Input: part model. Units: mm. Frame: model coordinates. A direction names the side the tool comes from. Round coordinates to 2 decimals unless told otherwise and drop trailing zeros. Loops run counter-clockwise (first coordinate to the right, second up) from the corner with the lowest first, then second, coordinate; pieces in that order, holes last.
1) Ray query, line 1 along Z through (x, y) = (6, 1) (3 decimals); line 2 along X through (y, z) = (2.45, -4). Return the intervals inside material, ascending.
2) Draft query along X for faces 1 (the face through (-14.676, 2.535, 12.768)), 2 (the face through (19.378, 2.535, -1.703)), 3 (the face through (1.792, 1.014, -4.858)). Return one class per face: pulls with the +X half, pulls with the -X half, needs draft (parallel to the pull), parting line crosses it, or undercut.
3) Section A-A, the plane z = 6. Return loops of the section in (x, y) (3 decimals), and give its area (3 significant figures).
4) First-contact query: pin 1 (3.5 mm diameter, centred on x = 0, z = 0, fed in from +Y); pin 2 (7 mm diameter, centred on x = -6, z = 0, fed in from +Y). Flat tips, straight axial feed; report the tip coordinate or a pass-through.
5) Access query for faces 4 (the face through (12.768, 2.535, 14.676)), 5 (the face through (7.55, 2.54, -17.87)), 6 (the face through (18.956, 2.535, 4.369)), 7 (the face through (-18.89, 2.54, 4.4)), 8 (the face through (-2.17, 3.52, 9.76)). Directions: +Z, -Z, +X, -X, +Y, -Y. A direction counts if a zero-diameter tool reaches every point of the face in a straight line with its end or side. Return the directions, or none.
6) Section C-C, the plane x = 16. Return loops of the section in (y, z), and give its area (3 significant figures).
7) Section B-B, the plane x = 6. Return loops of the section in (y, z) (3 decimals), and give its area (3 significant figures).
Autodesk Inventor part; units mm, degrees
ref_plane "YZ Plane" through (0, 0, 0) normal (1, 0, 0) x (0, 1, 0)
ref_plane "XZ Plane" through (0, 0, 0) normal (0, 1, 0) x (-1, 0, 0)
ref_plane "XY Plane" through (0, 0, 0) normal (0, 0, 1) x (1, 0, 0)
sketch "Sketch1" plane through (0, 0, 0) normal (0, 1, 0) x (-1, 0, 0)
  circle A0 centre (0, 0) radius 17.5
  dimension "d0" = 35
extrude "Extrusion1" add sketch "Sketch1" along normal blind 5
sketch "Sketch2" plane through (0, 5, 0) normal (0, 1, 0) x (1, 0, 0)
  circle A0 centre (0, 0) radius 10
  dimension "d3" = 20
extrude "Extrusion2" cut sketch "Sketch2" against normal blind 3
sketch "Sketch3" plane through (0, 2, 0) normal (0, 1, 0) x (1, 0, 0)
  circle A0 centre (-6, 0) radius 2.125
  circle A1 centre (-6, 0) radius 2.125
  point P0 (0, 0)
  dimension "d7" = 4.25
extrude "Extrusion3" cut sketch "Sketch3" against normal through all
pattern_circular "Circular Pattern1" count 4 over 360 about axis through (0, 5, 0) along (0, -1, 0) of "Extrusion3"
sketch "Sketch4" plane through (0, 2, 0) normal (0, 1, 0) x (1, 0, 0)
  circle A0 centre (0, 0) radius 2.125
  dimension "d13" = 4.25
extrude "Extrusion4" cut sketch "Sketch4" against normal blind 1
sketch "Sketch6" plane through (0, 5, 0) normal (0, 1, 0) x (1, 0, 0)
  arc A0 (5.4078, 16.6435) -> (0, 17.5) centre (0, 0) ccw
  line L0 (0, 0) -> (5.4078, 16.6435) construction
  line L1 (0, 0) -> (0, 17.5) construction
  line L2 (0, 0) -> (4.3015, 27.1585)
  line L3 (0, 0) -> (27.497, 0) construction
  arc A1 (5.4078, 16.6435) -> (0, 17.5) centre (0, 0) ccw
  dimension "d16" = 18
  dimension "d17" = 81
sketch "Sketch7" plane through (0, 5, 0) normal (0, 1, 0) x (1, 0, 0)
  circle A0 centre (0, 0) radius 17.5
  arc A1 (5.4078, 16.6435) -> (0, 17.5) centre (0, 0) ccw
  line L0 (0, 0) -> (5.4078, 16.6435) construction
  line L1 (0, 0) -> (0, 17.5) construction
  line L2 (0, 0) -> (4.2807, 27.027)
  line L3 (0, 0) -> (27.3639, 0) construction
  line L4 (0, 17.5) -> (3.3584, 21.2042)
  line L5 (3.3584, 21.2042) -> (5.4078, 16.6435)
  dimension "d18" = 18
  dimension "d19" = 81
  dimension "d20" = 5
extrude "Extrusion5" add sketch "Sketch7" against normal blind 5 contours A0 L2 L5 | L4 L2 A0
pattern_circular "Circular Pattern2" count 20 over 360 about axis through (0, 0, 0) along (0, 1, 0) of "Extrusion5"
properties part number "SmallGear"
Final values:
1. line 1: z = -16.983 to -2.125, 2.125 to 16.983
1. line 2: x = -19.78 to -9.17, 9.17 to 19.78
2. face 1: pulls with the -X half
2. face 2: pulls with the +X half
2. face 3: undercut
3. outline: (-16.983, 0) - (-2.125, 0) - (-2.125, 2) - (-8, 2) - (-8, 5) - (-16.983, 5) - close; (2.125, 0) - (16.983, 0) - (16.983, 5) - (8, 5) - (8, 2) - (2.125, 2) - close
3. area: 113 mm2
4. pin 1: stops at y = 1
4. pin 2: stops at y = 2
5. face 4: +Z, +Y, -Y
5. face 5: -Z, +Y, -Y
5. face 6: +X, +Y, -Y
5. face 7: -X, +Y, -Y
5. face 8: +Y
6. outline: (0, -10.09) - (5, -10.09) - (5, 10.09) - (0, 10.09) - close
6. area: 101 mm2
7. outline: (0, -16.983) - (5, -16.983) - (5, -8) - (2, -8) - (2, -2.125) - (0, -2.125) - close; (0, 2.125) - (2, 2.125) - (2, 8) - (5, 8) - (5, 16.983) - (0, 16.983) - close
7. area: 113 mm2
